```python
from build123d import *

# Parameters (mm, degrees)
F0_W     = 63.5
F0_H     = 15.875
F0_R     = 2.38125
F1_DEPTH = 3.175
F2_DEPTH = 4.7625
F3_T     = -1.5875
F4_R     = 3.175
F4_R_2   = 2.38125
F5_DEPTH = 1.5875


with BuildPart() as f1:
    # F0 (on Top) → F1 (new body)
    with BuildSketch(Plane.XY):
        with Locations((15.875, -3.96875)):
            Rectangle(F0_W, F0_H)
        with Locations((-11.90625, -7.9375)):
            Circle(F0_R, mode=Mode.SUBTRACT)
        with Locations((-3.96875, -7.9375)):
            Circle(F0_R, mode=Mode.SUBTRACT)
        with Locations((3.96875, -7.9375)):
            Circle(F0_R, mode=Mode.SUBTRACT)
        with Locations((11.90625, -7.9375)):
            Circle(F0_R, mode=Mode.SUBTRACT)
        with Locations((19.84375, -7.9375)):
            Circle(F0_R, mode=Mode.SUBTRACT)
        with Locations((27.78125, -7.9375)):
            Circle(F0_R, mode=Mode.SUBTRACT)
        with Locations((35.71875, -7.9375)):
            Circle(F0_R, mode=Mode.SUBTRACT)
        with Locations((43.65625, -7.9375)):
            Circle(F0_R, mode=Mode.SUBTRACT)
        with Locations((-11.90625, 0)):
            Circle(F0_R, mode=Mode.SUBTRACT)
        with Locations((-3.96875, 0)):
            Circle(F0_R, mode=Mode.SUBTRACT)
        with Locations((3.96875, 0)):
            Circle(F0_R, mode=Mode.SUBTRACT)
        with Locations((11.90625, 0)):
            Circle(F0_R, mode=Mode.SUBTRACT)
        with Locations((19.84375, 0)):
            Circle(F0_R, mode=Mode.SUBTRACT)
        with Locations((27.78125, 0)):
            Circle(F0_R, mode=Mode.SUBTRACT)
        with Locations((35.71875, 0)):
            Circle(F0_R, mode=Mode.SUBTRACT)
        with Locations((43.65625, 0)):
            Circle(F0_R, mode=Mode.SUBTRACT)
    extrude(amount=F1_DEPTH)

    # F0 (on Top) → F2 (join)
    with BuildSketch(Plane.XY):
        with Locations((-11.90625, 0)):
            Circle(F0_R)
        with Locations((-11.90625, -7.9375)):
            Circle(F0_R)
        with Locations((-3.96875, -7.9375)):
            Circle(F0_R)
        with Locations((-3.96875, 0)):
            Circle(F0_R)
        with Locations((3.96875, 0)):
            Circle(F0_R)
        with Locations((3.96875, -7.9375)):
            Circle(F0_R)
        with Locations((11.90625, -7.9375)):
            Circle(F0_R)
        with Locations((11.90625, 0)):
            Circle(F0_R)
        with Locations((19.84375, 0)):
            Circle(F0_R)
        with Locations((27.78125, 0)):
            Circle(F0_R)
        with Locations((27.78125, -7.9375)):
            Circle(F0_R)
        with Locations((19.84375, -7.9375)):
            Circle(F0_R)
        with Locations((35.71875, 0)):
            Circle(F0_R)
        with Locations((43.65625, 0)):
            Circle(F0_R)
        with Locations((43.65625, -7.9375)):
            Circle(F0_R)
        with Locations((35.71875, -7.9375)):
            Circle(F0_R)
    extrude(amount=F2_DEPTH)

    # F3
    f3_openings = [f1.faces().sort_by_distance(p)[0] for p in [
        (15.875, -3.96875, 0),
    ]]
    offset(amount=F3_T, openings=f3_openings, kind=Kind.INTERSECTION)

    # F4 (on face) → F5 (join)
    with BuildSketch(Plane(origin=(0, 0, 1.5875), x_dir=(1, 0, 0), z_dir=(0, 0, -1))):
        with BuildLine():
            ThreePointArc((-4.7625, 3.96875), (-6.7224801022, 6.9020675157), (-10.1825640303, 6.2138140303))
            Line((-10.1825640303, 6.2138140303), (-9.6212980227, 5.6525480227))
            ThreePointArc((-9.6212980227, 5.6525480227), (-7.0262350767, 6.1687381368), (-5.55625, 3.96875))
            ThreePointArc((-5.55625, 3.96875), (-5.7375118632, 3.0574850767), (-6.2537019773, 2.2849519773))
            Line((-6.2537019773, 2.2849519773), (-5.6924359697, 1.7236859697))
            ThreePointArc((-5.6924359697, 1.7236859697), (-5.0041824843, 2.7537301022), (-4.7625, 3.96875))
        make_face()
        with BuildLine():
            Line((-9.6212980227, 5.6525480227), (-10.1825640303, 6.2138140303))
            ThreePointArc((-10.1825640303, 6.2138140303), (-10.1825640303, 1.7236859697), (-5.6924359697, 1.7236859697))
            Line((-5.6924359697, 1.7236859697), (-6.2537019773, 2.2849519773))
            ThreePointArc((-6.2537019773, 2.2849519773), (-9.6212980227, 2.2849519773), (-9.6212980227, 5.6525480227))
        make_face()
        with Locations((0, 3.96875)):
            Circle(F4_R)
        with Locations((0, 3.96875)):
            Circle(F4_R_2, mode=Mode.SUBTRACT)
        with Locations((7.9375, 3.96875)):
            Circle(F4_R)
        with Locations((7.9375, 3.96875)):
            Circle(F4_R_2, mode=Mode.SUBTRACT)
        with Locations((15.875, 3.96875)):
            Circle(F4_R)
        with Locations((15.875, 3.96875)):
            Circle(F4_R_2, mode=Mode.SUBTRACT)
        with Locations((23.8125, 3.96875)):
            Circle(F4_R)
        with Locations((23.8125, 3.96875)):
            Circle(F4_R_2, mode=Mode.SUBTRACT)
        with Locations((31.75, 3.96875)):
            Circle(F4_R)
        with Locations((31.75, 3.96875)):
            Circle(F4_R_2, mode=Mode.SUBTRACT)
        with Locations((39.6875, 3.96875)):
            Circle(F4_R)
        with Locations((39.6875, 3.96875)):
            Circle(F4_R_2, mode=Mode.SUBTRACT)
    extrude(amount=F5_DEPTH)


solid = f1.part
```
Source: CAD feature listing. Evaluate the final solid. Frame: model axes, mm. A direction names the side the tool comes from. Coordinates: 2 decimals unless noted, no trailing zeros. Order: outer loops, then holes, each group sorted by start corner. A loop starts at its lowest first (then second) coordinate and runs counter-clockwise, first axis right, second up. Notation, with made-up numbers: M -28.5,-31 L 6.5,-31 A16 ccw 6.5,-8 Z; hole C 76,78 d1. An arc over 180 degrees is marked long. Write each question's results on one line, items separated by ' | '. Start each with the question number.
1) Contact query for flat-ended pins moving along their axis: pin 1 Ø1.7 at (x, y) = (4, -8) entering from -Z; pin 2 Ø1 at (x, y) = (43.66, 0) entering from -Z (3 decimals). Output: stop coordinate, or through.
2) Draft query along X for faces 1 (the face through (20.64, -4.11, 0.8)), 2 (the face through (36, -8, 4.762)), 3 (the face through (-0.31, -6.33, 0.8)), 4 (the face through (-15.875, -4, 2)). Return one class per face: released by +X, released by -X, zero draft, split by the parting line, or undercut.
3) Section query A-A (z = 0.95). Give the number of separate pieces and of enclosed holes in the cut face, plus the area to 3 significant figures.
4) Line query: line 1 (Y direction, x = -8, z = 1.3); line 2 (Y direction, x = -12.5, z = 1.3); line 3 (X direction, y = -9.5, z = 0.4) (1 decimal). Output: solid intervals per line, ascending. Write a range as from..to.
5) Access query for faces 5 (the face through (15, -4, 3.175)), 6 (the face through (15, -10.319, 1)), 7 (the face through (-12, 0, 4.762)). Directions: +Z, -Z, +X, -X, +Y, -Y. A direction counts if a zero-diameter tool reaches every point of the face in a straight line with its end or side. Return the directions, or none.
6) Section query C-C (x = 8). Return the cut outline in (y, z) (1 decimal), plus the area to 3 significant figures.
Answers:
1) pin 1: stops at z = 1.59 | pin 2: stops at z = 3.175
2) face 1: undercut | face 2: zero draft | face 3: undercut | face 4: released by -X
3) separate pieces: 8 | enclosed holes: 8 | area: 339 mm^2
4) line 1: y = -11.91..-10.32, -7.14..-6.35, -1.59..-0.79, 2.38..3.97 | line 2: y = -11.91..-10.32, 2.38..3.97 | line 3: x = -15.9..-14.3, 46..47.6
5) face 5: +Z | face 6: -Z | face 7: +Z, +X, -X, +Y, -Y
6) outline: M -11.9,0 L -10.3,0 L -10.3,1.6 L -7.1,1.6 L -7.1,0 L -6.3,0 L -6.3,1.6 L -1.6,1.6 L -1.6,0 L -0.8,0 L -0.8,1.6 L 2.4,1.6 L 2.4,0 L 4,0 L 4,3.2 L -11.9,3.2 Z | area: 32.8 mm^2
